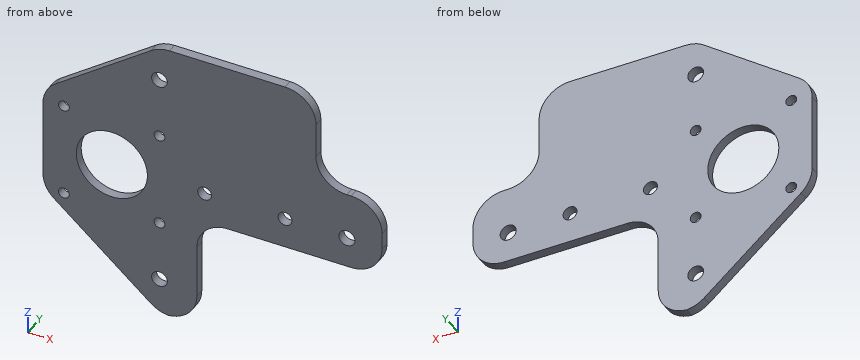
Autodesk Inventor part; units mm, degrees
ref_plane "YZ Plane" through (0, 0, 0) normal (1, 0, 0) x (0, 1, 0)
ref_plane "XZ Plane" through (0, 0, 0) normal (0, 1, 0) x (-1, 0, 0)
ref_plane "XY Plane" through (0, 0, 0) normal (0, 0, 1) x (1, 0, 0)
sketch "Sketch1" plane through (0, 0, 0) normal (0, 1, 0) x (-1, 0, 0)
  line L0 (-40.9159, 0.459) -> (-78.26, 0.459)
  line L1 (-109.64, -41.041) -> (-109.64, -46.541)
  line L2 (-39.76, -94.041) -> (-41.3348, -94.041)
  line L3 (0, -57.4156) -> (0, -32.0844)
  circle A0 centre (-22.26, -46.541) radius 11.5
  line L4 (-3.5248, -65.0361) -> (-34.8596, -91.6615)
  line L5 (-4.1082, -24.0044) -> (-35.0241, -1.461)
  line L6 (-49.76, -84.041) -> (-49.76, -66.541)
  line L7 (-59.76, -56.541) -> (-99.64, -56.541)
  line L8 (-98.26, -31.041) -> (-99.64, -31.041)
  line L9 (-88.26, -9.541) -> (-88.26, -21.041)
  arc A1 (-3.5248, -65.0361) -> (0, -57.4156) centre (-10, -57.4156) ccw
  arc A2 (0, -32.0844) -> (-4.1082, -24.0044) centre (-10, -32.0844) ccw
  arc A3 (-35.0241, -1.461) -> (-40.9159, 0.459) centre (-40.9159, -9.541) ccw
  arc A4 (-78.26, 0.459) -> (-88.26, -9.541) centre (-78.26, -9.541) ccw
  arc A5 (-98.26, -31.041) -> (-88.26, -21.041) centre (-98.26, -21.041) ccw
  arc A6 (-99.64, -31.041) -> (-109.64, -41.041) centre (-99.64, -41.041) ccw
  arc A7 (-109.64, -46.541) -> (-99.64, -56.541) centre (-99.64, -46.541) ccw
  arc A8 (-49.76, -66.541) -> (-59.76, -56.541) centre (-59.76, -66.541) ccw
  arc A9 (-49.76, -84.041) -> (-39.76, -94.041) centre (-39.76, -84.041) ccw
  arc A10 (-41.3348, -94.041) -> (-34.8596, -91.6615) centre (-41.3348, -84.041) ccw
  point P0 (0, 0)
  point P1 (0, -62.041)
  point P2 (-37.66, -94.041)
  point P3 (0, -27)
  point P4 (-37.6572, 0.459)
  point P5 (0, -44.75)
  point P6 (-40.5474, -94.01)
  dimension "d0" = 94.5
  dimension "d1" = 109.64
  dimension "d2" = 23
  dimension "d3" = 47
  dimension "d4" = 22.26
  dimension "d5" = 37.66
  dimension "d6" = 32
  dimension "d7" = 37.66
  dimension "d8" = 27
  dimension "d11" = 57
  dimension "d12" = 49.76
  dimension "d15" = 25.5
  dimension "d16" = 88.26
  dimension "d17" = 10
extrude "Extrusion1" add sketch "Sketch1" along normal blind 3 contours A3 L5 A2 L3 A1 L4 A10 A9 L6 A8 L7 A7 L1 A6 L8 A5 L9 A4 L0
sketch "Sketch2" plane through (0, 3, 0) normal (0, 1, 0) x (1, 0, 0)
  line L0 (40.9159, -0.459) -> (78.26, -0.459)
  line L1 (0, 57.4156) -> (0, 32.0844)
  point P0 (0, 0)
  point P1 (6.76, 62.041)
  point P2 (37.66, 62.041)
  point P3 (37.66, 31.041)
  point P4 (6.76, 31.041)
  dimension "d20" = 31.5
  dimension "d21" = 37.66
  dimension "d22" = 62.5
  dimension "d23" = 6.76
hole "Hole1" at (6.76, 3, -62.041) at (37.66, 3, -62.041) at (37.66, 3, -31.041) at (6.76, 3, -31.041) direction (0, -1, 0) diameter 3.5 end through all
sketch "Sketch3" plane through (0, 3, 0) normal (0, 1, 0) x (1, 0, 0)
  line L0 (40.9159, -0.459) -> (78.26, -0.459)
  line L1 (0, 57.4156) -> (0, 32.0844)
  point P0 (0, 0)
  point P1 (37.66, 82.041)
  point P2 (37.66, 11.041)
  dimension "d31" = 82.5
  dimension "d32" = 11.5
  dimension "d33" = 37.66
hole "Hole2" at (37.66, 3, -82.041) at (37.66, 3, -11.041) direction (0, -1, 0) diameter 5.1 end through all
sketch "Sketch4" plane through (0, 3, 0) normal (0, 1, 0) x (1, 0, 0)
  line L0 (40.9159, -0.459) -> (78.26, -0.459)
  line L1 (0, 57.4156) -> (0, 32.0844)
  point P0 (0, 0)
  point P1 (52.26, 46.541)
  point P2 (78.26, 46.541)
  dimension "d41" = 47
  dimension "d42" = 52.26
  dimension "d43" = 78.26
hole "Hole3" at (52.26, 3, -46.541) at (78.26, 3, -46.541) direction (0, -1, 0) diameter 4.5 end through all
sketch "Sketch5" plane through (0, 3, 0) normal (0, 1, 0) x (1, 0, 0)
  line L0 (0, 57.4156) -> (0, 32.0844)
  line L1 (40.9159, -0.459) -> (78.26, -0.459)
  point P0 (0, 0)
  point P1 (98.26, 46.541)
  dimension "d51" = 98.26
  dimension "d52" = 47
hole "Hole4" at (98.26, 3, -46.541) direction (0, -1, 0) diameter 5.2 end through all
properties part number "X Motor Bracket" material "Aluminum 6061"
Verification items for the finished model (mm, model axes). Round coordinates to 2 decimals unless told otherwise and drop trailing zeros. Order: outer loops, then holes, each group sorted by start corner. A loop starts at its lowest first (then second) coordinate and runs counter-clockwise, first axis right, second up. Notation, with made-up numbers: (14.25, 53) -> (36.25, 53) arc R29 cw to (36.25, 91) -> close; hole circle Ø11 at (26, -32.75). An arc over 180 degrees is marked (long way). Put each result on its own line as item: value.
1) Section check C-C (x = 22.26). Record the cut outline in (y, z).
Final values:
outline: (0, -80.96) -> (3, -80.96) -> (3, -58.04) -> (0, -58.04) -> close; (0, -35.04) -> (3, -35.04) -> (3, -10.77) -> (0, -10.77) -> close
2) Section check A-A (y = 1.9). Give the number of separate pieces and of enclosed holes in the cut face, then the cut area to 3 significant figures.
Final values:
separate pieces: 1
enclosed holes: 10
area: 5,720 mm^2
3) Depth check by flat-ended pin: pin 1 (2.5 mm diameter, centred on x = 52.26, z = -46.541, fed in from -Y); pin 2 (0.7 mm diameter, centred on x = 99, y = 2, fed in from +Z); pin 3 (0.9 mm diameter, centred on x = 82, y = 1.5, fed in from -Z). Enter the tip coordinate at first touch or a pass-through.
Final values:
pin 1: passes through
pin 2: stops at z = -31.04
pin 3: stops at z = -56.54
4) Section check D-D (x = 6.76). Record the cut outline in (y, z).
Final values:
outline: (0, -67.79) -> (3, -67.79) -> (3, -63.79) -> (0, -63.79) -> close; (0, -60.29) -> (3, -60.29) -> (3, -32.79) -> (0, -32.79) -> close; (0, -29.29) -> (3, -29.29) -> (3, -22.07) -> (0, -22.07) -> close
5) Material ranges on line 1 (X direction, y = 0.4, z = -45); line 2 (X direction, y = 1.05, z = -9.5); line 3 (Z direction, x = 78, y = 2.5), recorded low to high.
Final values:
line 1: x = 0 to 10.86, 33.66 to 50.62, 53.9 to 76.62, 79.9 to 96.17, 100.35 to 109.64
line 2: x = 24 to 35.63, 39.69 to 88.26
line 3: z = -56.54 to -48.78, -44.31 to 0.46
6) Section check B-B (x = 37.66). Record the cut outline in (y, z), then the cut area to 3 significant figures.
Final values:
outline: (0, -93.34) -> (3, -93.34) -> (3, -84.59) -> (0, -84.59) -> close; (0, -79.49) -> (3, -79.49) -> (3, -63.79) -> (0, -63.79) -> close; (0, -60.29) -> (3, -60.29) -> (3, -32.79) -> (0, -32.79) -> close; (0, -29.29) -> (3, -29.29) -> (3, -13.59) -> (0, -13.59) -> close; (0, -8.49) -> (3, -8.49) -> (3, -0.09) -> (0, -0.09) -> close
area: 228 mm^2
